For this review, use the dimensioned drawing (mm, ordinates from the lowest corner) and the shaded views. Round coordinates to 2 decimals unless told otherwise and drop trailing zeros. Loops run counter-clockwise (first coordinate to the right, second up) from the corner with the lowest first, then second, coordinate; pieces in that order, holes last. Notation, with made-up numbers: (-24.5, -34.75) -> (31.5, -34.75) arc R21 ccw to (31.5, -7.75) -> close; hole circle Ø4 at (1, 56). An arc over 180 degrees is marked (long way). Answer as CSV lines item,"result". Start each with the question number.
(1) Take a section at D-D, the plane y = 18. Write out the cut boundary in (x, z).
(2) Take a section at C-C, the plane x = 13.5. Write out the cut boundary in (y, z).
(3) To check wall thickness, follow line 1 (X direction, y = 3.5, z = 0.15); line 2 (Y direction, x = 39.5, z = 0.6) (1 decimal); line 3 (Y direction, x = 33, z = 1.05). State the ranges of each line that lie inside material, in increasing order. Write a range as from..to.
(4) Take a section at A-A, the plane y = 4.25. Write out the cut boundary in (x, z), and give its area (3 significant figures).
(5) Take a section at B-B, the plane z = 0.6. Write out the cut boundary in (x, y), and give its area (3 significant figures).
(6) For P1, Ø1, axis at x = 69, z = 1, coming from the -Y side; P2, Ø0.6, axis at y = 3, z = 1, coming from the -X side; P3, Ø1, axis at x = 78, z = 1, coming from the -Y side, all flat-tipped, find the tip position at first contact; note any pin that passes through.
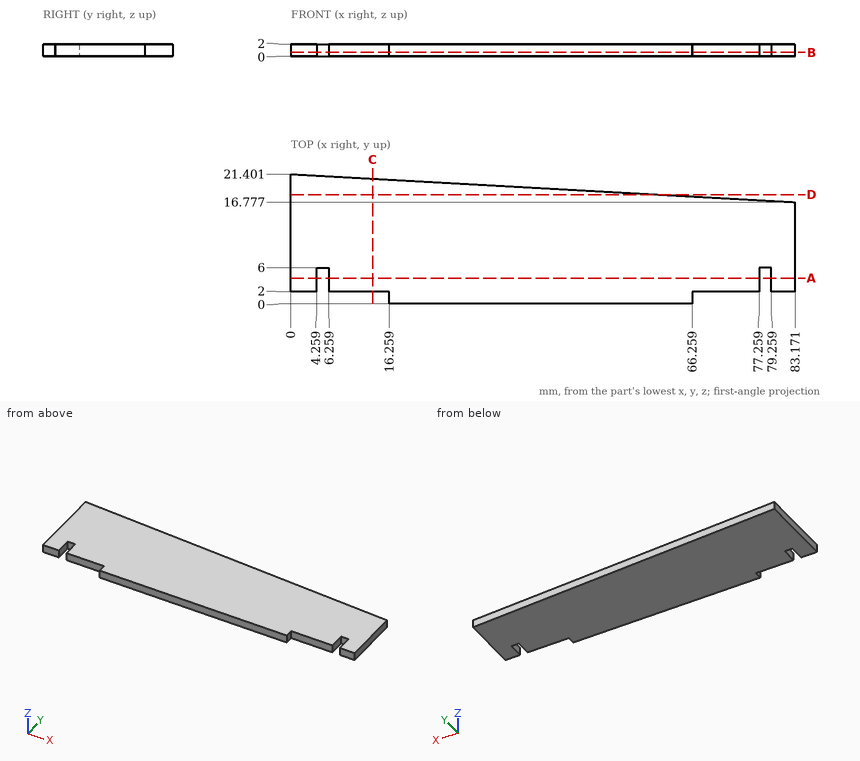
The answers:
1,outline,"(0, 0) -> (61.17, 0) -> (61.17, 2) -> (0, 2) -> close"
2,outline,"(2, 0) -> (20.65, 0) -> (20.65, 2) -> (2, 2) -> close"
3,line 1,"0..4.26, 6.26..77.26, 79.26..83.17"
3,line 2,"0..19.2"
3,line 3,"0..19.57"
4,outline,"(0, 0) -> (4.26, 0) -> (4.26, 2) -> (0, 2) -> close; (6.26, 0) -> (77.26, 0) -> (77.26, 2) -> (6.26, 2) -> close; (79.26, 0) -> (83.17, 0) -> (83.17, 2) -> (79.26, 2) -> close"
4,area,"158 mm²"
5,outline,"(0, 2) -> (4.26, 2) -> (4.26, 6) -> (6.26, 6) -> (6.26, 2) -> (16.26, 2) -> (16.26, 0) -> (66.26, 0) -> (66.26, 2) -> (77.26, 2) -> (77.26, 6) -> (79.26, 6) -> (79.26, 2) -> (83.17, 2) -> (83.17, 16.78) -> (0, 21.4) -> close"
5,area,"1,510 mm²"
6,P1,"y = 2"
6,P2,"x = 0"
6,P3,"y = 6"
